Here's the drawing with two shaded views (mm, measured from the low corner). I have some questions. Give positions to 0.01 mm unless a question says otherwise; leave off trailing zeros. Order: outer loops, then holes, each group sorted by start corner. A loop starts at its lowest first (then second) coordinate and runs counter-clockwise, first axis right, second up. Notation, with made-up numbers: M -38.5,15.25 L 0.5,15.25 A35 cw 0.5,48.25 Z; hole C 1,-30 d4. An arc over 180 degrees is marked long. One line per question, with ' | ' between items. Start each with the question number.
1) Please list where these lines run through material, in increasing order: line 1 along X through (y, z) = (2.1, 5); line 2 along X through (y, z) = (1.5, 46); line 3 along Z through (x, y) = (48, 1.65). Write a range as [from, to].
2) I'm going to push a flat-ended pin straight in: pin 1 Ø1.9 at (x, z) = (15, 65) entering from +Y. Where does the tip first touch, or does it pass through?
3) If we section it at A-A, the plane z = 75: Please give me the cut outline in (x, y) (3 decimals), plus the area to 3 significant figures.
4) If we section it at B-B, the plane x = 5: State how many separate pieces and enclosed holes the cut face has, plus the area to 3 significant figures.
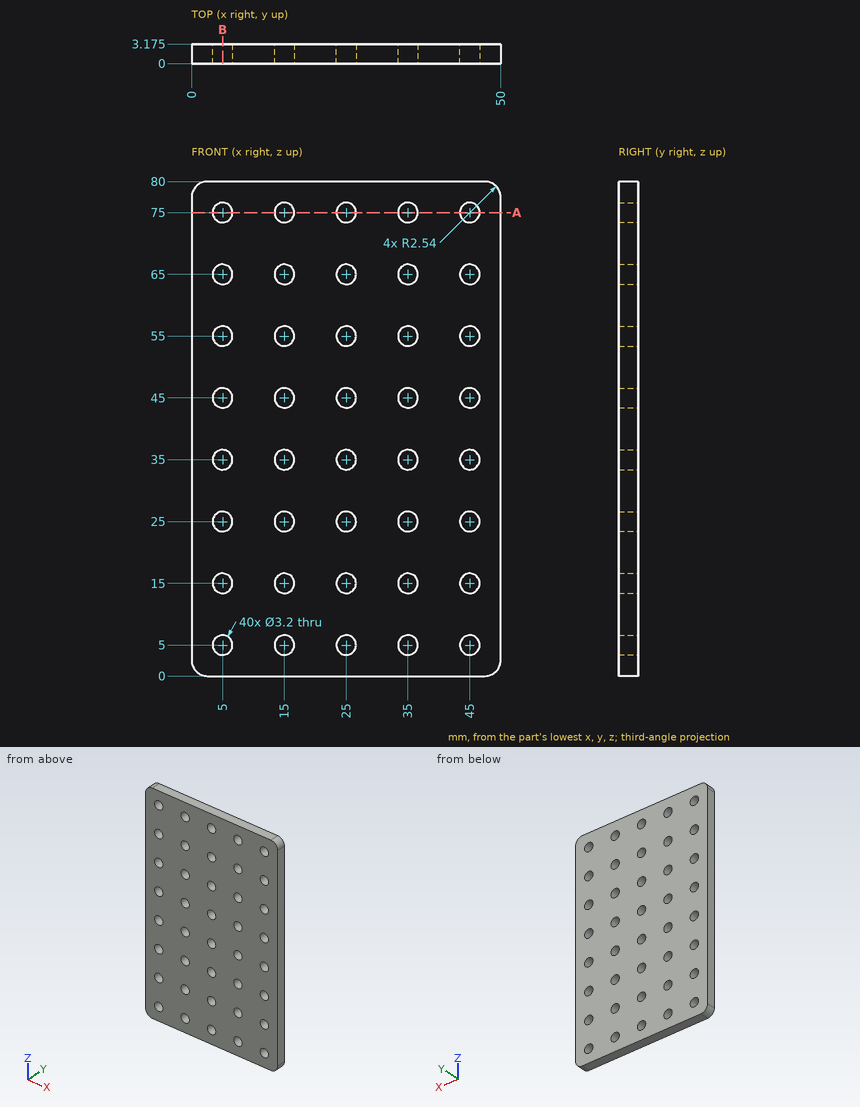
Results found:
1) line 1: x = [0, 3.4], [6.6, 13.4], [16.6, 23.4], [26.6, 33.4], [36.6, 43.4], [46.6, 50] | line 2: x = [0, 3.75], [6.25, 13.75], [16.25, 23.75], [26.25, 33.75], [36.25, 43.75], [46.25, 50] | line 3: z = [0.06, 79.94]
2) pin 1: passes through
3) outline: M 0,0 L 3.4,0 L 3.4,3.175 L 0,3.175 Z; M 6.6,0 L 13.4,0 L 13.4,3.175 L 6.6,3.175 Z; M 16.6,0 L 23.4,0 L 23.4,3.175 L 16.6,3.175 Z; M 26.6,0 L 33.4,0 L 33.4,3.175 L 26.6,3.175 Z; M 36.6,0 L 43.4,0 L 43.4,3.175 L 36.6,3.175 Z; M 46.6,0 L 50,0 L 50,3.175 L 46.6,3.175 Z | area: 108 mm²
4) separate pieces: 9 | enclosed holes: 0 | area: 173 mm²
